Source: CAD feature listing. Evaluate the final solid. Frame: model axes, mm. A direction names the side the tool comes from. Round coordinates to 2 decimals unless told otherwise and drop trailing zeros. Loops run counter-clockwise (first coordinate to the right, second up) from the corner with the lowest first, then second, coordinate; pieces in that order, holes last. Notation, with made-up numbers: (33.5, 43.25) -> (37.5, 43.25) arc R6 cw to (37.5, 54.25) -> close; hole circle Ø10 at (-6, 4). An arc over 180 degrees is marked (long way). Write item = value, one per line.
from build123d import *

# Parameters (mm, degrees)
BOSS_EXTRUDE1_DEPTH      = 20
BOSS_EXTRUDE1_DEPTH_BACK = 20
SKETCH1_R                = 60
SKETCH1_R_2              = 52
CUT_EXTRUDE1_DEPTH       = 20
CUT_EXTRUDE1_DEPTH_BACK  = 20


with BuildPart() as part:
    # Sketch1 → Boss-Extrude1 (new, two sides: drawn at the far end of the back side and taken through both)
    with BuildSketch(Plane.XY.offset(-BOSS_EXTRUDE1_DEPTH_BACK)):
        Circle(SKETCH1_R)
        Circle(SKETCH1_R_2, mode=Mode.SUBTRACT)
    extrude(amount=BOSS_EXTRUDE1_DEPTH + BOSS_EXTRUDE1_DEPTH_BACK)

    # Sketch2 → Cut-Extrude1 (cut, two sides: drawn at the far end of the back side and taken through both)
    with BuildSketch(Plane.XY.offset(-CUT_EXTRUDE1_DEPTH_BACK)):
        Polygon((51.978001404, -1.512405375), (56.465581727, -1.512405375), (56.465581727, 1.971821564), (51.962601164, 1.971821564), align=None)
    extrude(amount=CUT_EXTRUDE1_DEPTH + CUT_EXTRUDE1_DEPTH_BACK, mode=Mode.SUBTRACT)


solid = part.part
1. Line query: probe 1 along Y at (x, z) = (0, 9.5); probe 2 along X at (y, z) = (-36.5, -16); probe 3 along Y at (x, z) = (-47, 18.5). Output: solid intervals per line, ascending. Write a range as from..to.
Evaluation:
probe_1 = -60..-52, 52..60
probe_2 = -47.62..-37.04, 37.04..47.62
probe_3 = -37.3..-22.25, 22.25..37.3
2. Section query A-A (x = 0). Return the cut outline in (y, z).
Evaluation:
outline = (-60, -20) -> (-52, -20) -> (-52, 20) -> (-60, 20) -> close; (52, -20) -> (60, -20) -> (60, 20) -> (52, 20) -> close
3. Section query B-B (y = 0). Return the cut outline in (x, z).
Evaluation:
outline = (-60, -20) -> (-52, -20) -> (-52, 20) -> (-60, 20) -> close; (56.47, -20) -> (60, -20) -> (60, 20) -> (56.47, 20) -> close
4. Mould query, pull axis Y, two halves, no side actions, for faces 3 (the face through (-59.94, 2.64, -0.28)), 4 (the face through (-51.96, 2.03, -0.28)), 5 (the face through (-49, 18, 20)). Classes: released by +Y, released by -Y, zero draft, split by the parting line, or undercut.
Evaluation:
face_3 = split by the parting line
face_4 = undercut
face_5 = zero draft
5. Set-up query: faces 1 (the face through (-49, 18, -20)), 2 (the face through (54, 1.972, 0)). Return all of +Z, -Z, +X, -X, +Y, -Y with unobstructed straight access to the full face (end or side cutting, diameter ignored); none if empty.
Evaluation:
face_1 = -Z, +X, -X, +Y, -Y
face_2 = +Z, -Z
6. Contact query for flat-ended pins moving along their axis: pin 1 Ø8 at (x, z) = (-38, 11) entering from -Y; pin 2 Ø2 at (x, z) = (7, -15.5) entering from +Y; pin 3 Ø3.5 at (x, z) = (53, -9.5) entering from +Y. Output: stop coordinate, or through.
Evaluation:
pin_1 = -49.44
pin_2 = 59.7
pin_3 = 31.2
7. Section query C-C (z = -6). Return the cut outline in (x, y), then the cut area to 3 significant figures.
Evaluation:
outline = circle Ø120 at (0, 0); hole (51.96, 1.97) arc R52 ccw (long way) to (51.98, -1.51) -> (56.47, -1.51) -> (56.47, 1.97) -> close
area = 2,800 mm²
